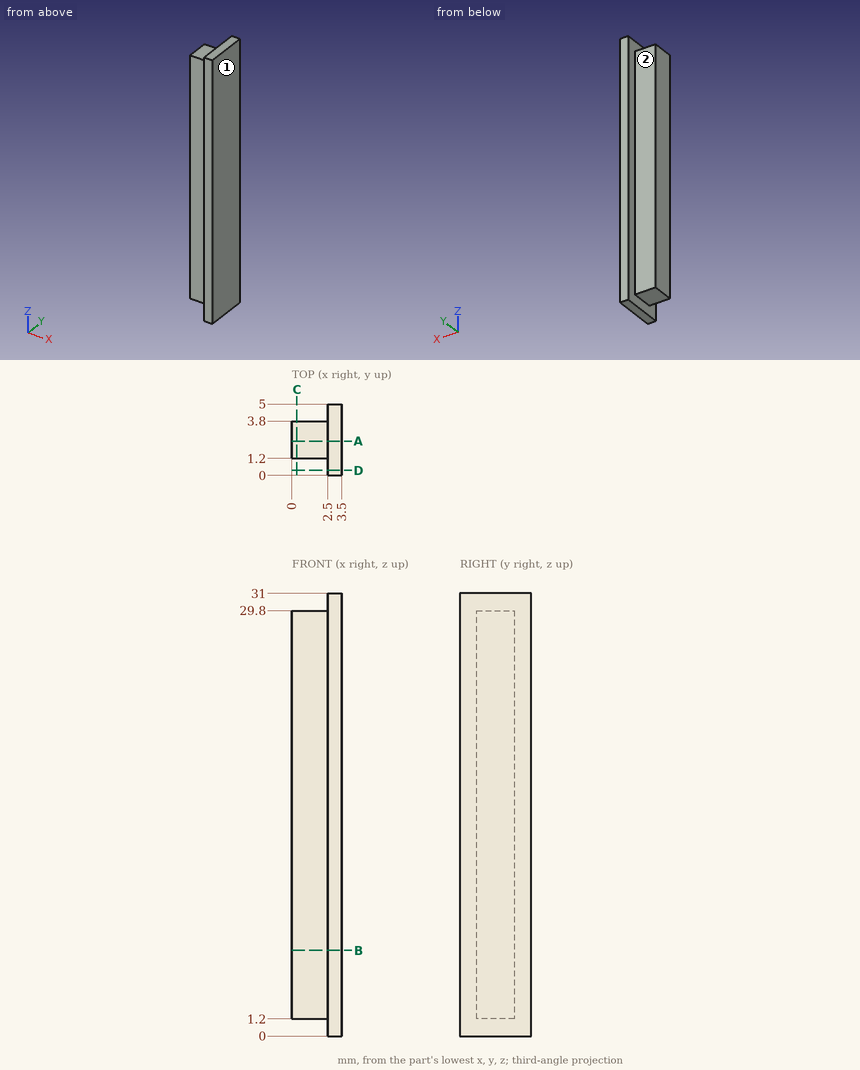
Print and shaded views of the part. All mm, measured from the part's lowest x, y and z. A direction names the side the tool comes from. Coordinates: 2 decimals unless noted, no trailing zeros. Loops run counter-clockwise (first coordinate to the right, second up) from the corner with the lowest first, then second, coordinate; pieces in that order, holes last. Notation, with made-up numbers: M -13,45.5 L 26,45.5 A16 cw 26,56.5 Z; hole C 58.5,88.25 d8. An arc over 180 degrees is marked long. Use a Markdown table: item, result. Add a question column.
Q1. Pin check, flat tips, straight feed: P1, Ø1.5, axis at x = 1.5, z = 4, coming from the -Y side; P2, Ø0.8, axis at x = 1.5, y = 2.5, coming from the +Z side. Stop position of each tip, or through.
Q2. Cut at A-A (y = 2.4). Write the cut outline in (x, z).
Q3. Which spindle directions (+Z, -Z, +X, -X, +Y, -Y) get a long thin tool onto all of the face, cutting with end or side? Do the marked faces 1 and 2. Say none if no direction does.
Q4. Probe L1, parallel to Z at x = 2.1, y = 2.55; L2, parallel to X at y = 4.45, z = 23; L3, parallel to Y at x = 1.3, z = 23. List the from-to ranges inside material, lowest first.
Q5. Cut at C-C (x = 0.35). Write the cut outline in (y, z), and give its area (3 significant figures).
Q6. Cut at D-D (y = 0.35). Write the cut outline in (x, z).
Q7. Cut at B-B (z = 6). Write the cut outline in (x, y).
Worked out:
| question | item | result |
|---|---|---|
| 1 | P1 | stops at y = 1.2 |
| 1 | P2 | stops at z = 29.8 |
| 2 | outline | M 0,1.2 L 2.5,1.2 L 2.5,0 L 3.5,0 L 3.5,31 L 2.5,31 L 2.5,29.8 L 0,29.8 Z |
| 3 | face 1 | +Z, -Z, +X, +Y, -Y |
| 3 | face 2 | +Z, -Z, -X, +Y |
| 4 | L1 | z = 1.2 to 29.8 |
| 4 | L2 | x = 2.5 to 3.5 |
| 4 | L3 | y = 1.2 to 3.8 |
| 5 | outline | M 1.2,1.2 L 3.8,1.2 L 3.8,29.8 L 1.2,29.8 Z |
| 5 | area | 74.4 mm2 |
| 6 | outline | M 2.5,0 L 3.5,0 L 3.5,31 L 2.5,31 Z |
| 7 | outline | M 0,1.2 L 2.5,1.2 L 2.5,0 L 3.5,0 L 3.5,5 L 2.5,5 L 2.5,3.8 L 0,3.8 Z |
